Design review of the part built by this model. Coordinates are the model's own, in mm. Coordinates: 2 decimals unless noted, no trailing zeros. Loops run counter-clockwise (first coordinate to the right, second up) from the corner with the lowest first, then second, coordinate; pieces in that order, holes last.
Q1. Wall thickness on probe 1 along Z at (x, y) = (58.5, 2.85) (3 decimals); probe 2 along Z at (x, y) = (-11.5, 2.4) (3 decimals); probe 3 along Z at (x, y) = (-68, 2.3) (3 decimals): over which ranges is each line inside the solid? List them lowest first.
Q2. Add section A-A on x = 91.5. Give the boundary of the cut face in (y, z) (3 decimals).
Q3. Add section B-B on y = 1.7. Give the number of separate pieces and of enclosed holes in the cut face, and give its area (3 significant figures).
Q4. For P1, Ø2, axis at x = 112.5, y = 2, coming from the -Z side (3 decimals), flat-tipped, find the tip position at first contact; note if it passes through.
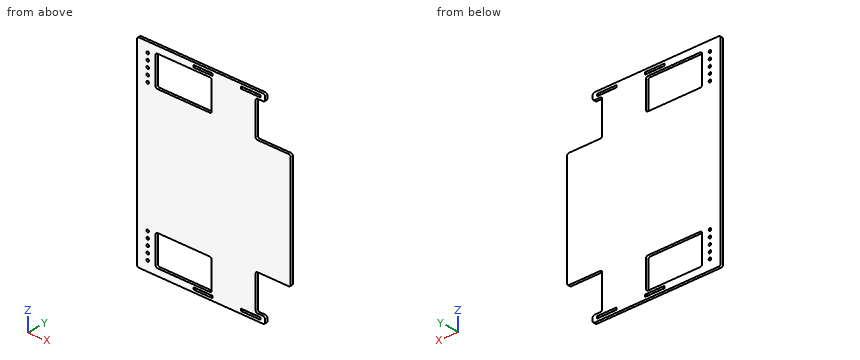
```python
from build123d import *

# Parameters (mm, degrees)
SKETCH1_R           = 2
SKETCH1_W           = 30.4
SKETCH1_H           = 3.35
SKETCH1_W_2         = 88
SKETCH1_H_2         = 48
BOSS_EXTRUDE1_DEPTH = 4
FILLET1_R           = 3


with BuildPart() as part:
    # Sketch1 → Boss-Extrude1 (new body)
    with BuildSketch(Plane(origin=(0, 0, 0), x_dir=(1, 0, 0), z_dir=(0, 1, 0))):
        Polygon((-112.8, 156.215), (-112.8, -156.215), (87.95, -156.215), (87.95, -145.555), (73.17, -145.555), (73.17, -89.625), (128.17, -89.625), (128.17, 89.625), (73.17, 89.625), (73.17, 145.555), (87.95, 145.555), (87.95, 156.215), align=None)
        with Locations(Location((-96, 140.715, 0), (0, 0, 270))):
            Circle(SKETCH1_R, mode=Mode.SUBTRACT)
        with Locations(Location((-96, 130.715, 0), (0, 0, 270))):
            Circle(SKETCH1_R, mode=Mode.SUBTRACT)
        with Locations(Location((-96, 120.715, 0), (0, 0, 270))):
            Circle(SKETCH1_R, mode=Mode.SUBTRACT)
        with Locations(Location((-96, 110.715, 0), (0, 0, 270))):
            Circle(SKETCH1_R, mode=Mode.SUBTRACT)
        with Locations(Location((-96, 100.715, 0), (0, 0, 270))):
            Circle(SKETCH1_R, mode=Mode.SUBTRACT)
        with Locations(Location((-96, -100.715, 0), (0, 0, 90))):
            Circle(SKETCH1_R, mode=Mode.SUBTRACT)
        with Locations(Location((-96, -110.715, 0), (0, 0, 90))):
            Circle(SKETCH1_R, mode=Mode.SUBTRACT)
        with Locations(Location((-96, -120.715, 0), (0, 0, 90))):
            Circle(SKETCH1_R, mode=Mode.SUBTRACT)
        with Locations(Location((-96, -130.715, 0), (0, 0, 90))):
            Circle(SKETCH1_R, mode=Mode.SUBTRACT)
        with Locations(Location((-96, -140.715, 0), (0, 0, 90))):
            Circle(SKETCH1_R, mode=Mode.SUBTRACT)
        with Locations((65.59, 150.74)):
            Rectangle(SKETCH1_W, SKETCH1_H, mode=Mode.SUBTRACT)
        with Locations((-39.71, 121.555)):
            Rectangle(SKETCH1_W_2, SKETCH1_H_2, mode=Mode.SUBTRACT)
        with Locations((-9.41, 150.74)):
            Rectangle(SKETCH1_W, SKETCH1_H, mode=Mode.SUBTRACT)
        with Locations((65.59, -150.74)):
            Rectangle(SKETCH1_W, SKETCH1_H, mode=Mode.SUBTRACT)
        with Locations((-9.41, -150.74)):
            Rectangle(SKETCH1_W, SKETCH1_H, mode=Mode.SUBTRACT)
        with Locations((-39.71, -121.555)):
            Rectangle(SKETCH1_W_2, SKETCH1_H_2, mode=Mode.SUBTRACT)
    extrude(amount=BOSS_EXTRUDE1_DEPTH)

    # Fillet1
    fillet1_edges = [part.edges().sort_by_distance(p)[0] for p in [
        (-83.71, 2, 97.555),
        (-83.71, 2, 145.555),
        (4.29, 2, 145.555),
        (4.29, 2, 97.555),
        (87.95, 2, -156.215),
        (87.95, 2, -145.555),
        (73.17, 2, -145.555),
        (73.17, 2, -89.625),
        (128.17, 2, -89.625),
        (128.17, 2, 89.625),
        (73.17, 2, 89.625),
        (73.17, 2, 145.555),
        (87.95, 2, 145.555),
        (87.95, 2, 156.215),
        (-112.8, 2, 156.215),
        (-112.8, 2, -156.215),
        (-83.71, 2, -145.555),
        (-83.71, 2, -97.555),
        (4.29, 2, -97.555),
        (4.29, 2, -145.555),
    ]]
    fillet(fillet1_edges, radius=FILLET1_R)


solid = part.part
```
Entries:
1. probe 1: z = -156.215 to -152.415, -149.065 to 149.065, 152.415 to 156.215
1. probe 2: z = -156.215 to -152.415, -149.065 to -145.555, -97.555 to 97.555, 145.555 to 149.065, 152.415 to 156.215
1. probe 3: z = -156.215 to -145.555, -97.555 to 97.555, 145.555 to 156.215
2. outline: (0, -89.625) - (4, -89.625) - (4, 89.625) - (0, 89.625) - close
3. separate pieces: 1
3. enclosed holes: 16
3. area: 59,300 mm2
4. P1: stops at z = -89.625
